CAD build for the part. Positions are in the model's coordinates, mm. Face numbers are marked on the shaded views. Give positions to 0.01 mm unless a question says otherwise; leave off trailing zeros. Order: outer loops, then holes, each group sorted by start corner. A loop starts at its lowest first (then second) coordinate and runs counter-clockwise, first axis right, second up.
```python
from build123d import *

# Parameters (mm, degrees)
F0_W     = 70.3723412007
F0_H     = 39.6034847945
F2_DEPTH = 9.5
F1_R     = 2.35
F3_DEPTH = 8


# Not quite as in the source:
# - the program builds the solid bodies; features that only make, move or delete a surface that nothing else refers to are left out


with BuildPart() as f2:
    # F0 (on Top) → F2 (new body)
    with BuildSketch(Plane.XY):
        with Locations((-25.7422635332, 26.3515496626)):
            Rectangle(F0_W, F0_H)
    extrude(amount=F2_DEPTH)

    # F1 (on face) → F3 (cut)
    with BuildSketch(Plane.XY):
        with BuildLine():
            ThreePointArc((-26.0081397088, 24.315958029), (-26.0169226605, 24.8283618655), (-26.0432611967, 25.3401636957))
            ThreePointArc((-26.0432611967, 25.3401636957), (-29.6543131579, 29.4708098057), (-30.4048881867, 34.9057496103))
            ThreePointArc((-30.4048881867, 34.9057496103), (-54.7680712155, 18.5828288025), (-26.0081397088, 24.315958029))
        make_face()
        with BuildLine():
            ThreePointArc((-18.4289942121, 24.2039844017), (-10.2782880331, 12.4173582289), (0.4453969671, 21.9232063115))
            ThreePointArc((0.4453969671, 21.9232063115), (0.1704350534, 24.2013451557), (-0.6386587183, 26.348642973))
            ThreePointArc((-0.6386587183, 26.348642973), (-4.6497239534, 27.6234855531), (-6.8365136406, 31.2195693659))
            ThreePointArc((-6.8365136406, 31.2195693659), (-9.2433206047, 31.4975310038), (-11.6428466394, 31.1624828835))
            ThreePointArc((-11.6428466394, 31.1624828835), (-14.0873300566, 26.758138344), (-18.4289942121, 24.2039844017))
        make_face()
        with BuildLine():
            ThreePointArc((-26.0432611967, 25.3401636957), (-22.3553467612, 23.9731105992), (-18.4289942121, 24.2039844017))
            ThreePointArc((-18.4289942121, 24.2039844017), (-15.9845107949, 28.6083289412), (-11.6428466394, 31.1624828835))
            ThreePointArc((-11.6428466394, 31.1624828835), (-11.436389736, 32.2945759735), (-11.3672378186, 33.4432609737))
            ThreePointArc((-11.3672378186, 33.4432609737), (-20.2088389756, 42.9901322485), (-30.4048881867, 34.9057496103))
            ThreePointArc((-30.4048881867, 34.9057496103), (-27.3555998695, 30.5189557333), (-26.0432611967, 25.3401636957))
        make_face()
        with Locations((-20.9422378186, 33.4432609737)):
            Circle(F1_R, mode=Mode.SUBTRACT)
        with BuildLine():
            ThreePointArc((-6.8365136406, 31.2195693659), (-3.2130730762, 29.4515061375), (-0.6386587183, 26.348642973))
            ThreePointArc((-0.6386587183, 26.348642973), (3.4064099368, 28.2070418834), (5.0577621814, 32.340958029))
            ThreePointArc((5.0577621814, 32.340958029), (-1.5054185479, 38.3144685099), (-6.8365136406, 31.2195693659))
        make_face()
        with BuildLine():
            ThreePointArc((-30.4048881867, 34.9057496103), (-29.6543131579, 29.4708098057), (-26.0432611967, 25.3401636957))
            ThreePointArc((-26.0432611967, 25.3401636957), (-27.3555998695, 30.5189557333), (-30.4048881867, 34.9057496103))
        make_face()
        with BuildLine():
            ThreePointArc((-11.6428466394, 31.1624828835), (-15.9845107949, 28.6083289412), (-18.4289942121, 24.2039844017))
            ThreePointArc((-18.4289942121, 24.2039844017), (-14.0873300566, 26.758138344), (-11.6428466394, 31.1624828835))
        make_face()
        with Locations((-20.9422378186, 33.4432609737)):
            Circle(F1_R)
        with BuildLine():
            ThreePointArc((-6.8365136406, 31.2195693659), (-4.6497239534, 27.6234855531), (-0.6386587183, 26.348642973))
            ThreePointArc((-0.6386587183, 26.348642973), (-3.2130730762, 29.4515061375), (-6.8365136406, 31.2195693659))
        make_face()
    extrude(amount=F3_DEPTH, mode=Mode.SUBTRACT)


solid = f2.part
```
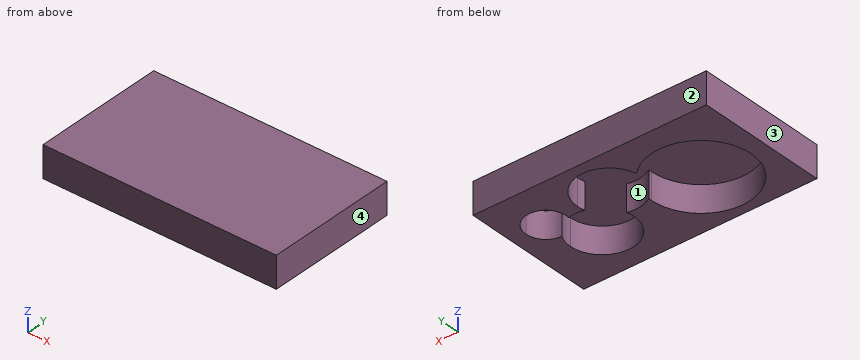
Item 1: Two-plate mould, pull along X, no slides. Class the marked faces 1, 2, 3 and 4: released by +X, released by -X, zero draft, split by the parting line, or undercut.
Item 2: Slice it at C-C (y = 41). Give the cut face in (x, z), and give its area (3 significant figures).
Item 3: Slice it at B-B (x = -43). Give the cut face in (y, z), and give its area (3 significant figures).
Item 4: Slice it at A-A (z = 1.75). Give the cut face in (x, y) (3 decimals), and give its area (3 significant figures).
Item 5: Wall check: L1, parallel to X at y = 25, z = 3; L2, parallel to X at y = 19, z = 0.5; L3, parallel to Z at x = -4, y = 28. Give the ranges that are in metal, low to high.
Item 6: Slice it at D-D (y = 16). Give the cut face in (x, z), and give its area (3 significant figures).
Item 7: Drop a flat-ended pin along its axis: pin 1 Ø1 at (x, y) = (-52.5, 26.5) entering from -Z. Give the stop position or say it passes through.
A:
1. face 1: undercut
1. face 2: zero draft
1. face 3: released by -X
1. face 4: released by +X
2. outline: (-60.93, 0) - (-26.82, 0) - (-26.82, 8) - (-15.06, 8) - (-15.06, 0) - (9.44, 0) - (9.44, 9.5) - (-60.93, 9.5) - close
2. area: 574 mm2
3. outline: (6.55, 0) - (9.5, 0) - (9.5, 8) - (39.13, 8) - (39.13, 0) - (46.15, 0) - (46.15, 9.5) - (6.55, 9.5) - close
3. area: 139 mm2
4. outline: (-60.928, 6.55) - (9.444, 6.55) - (9.444, 46.153) - (-60.928, 46.153) - close; hole (-30.405, 34.906) arc R14.951 ccw (long way) to (-26.043, 25.34) arc R9.575 ccw to (-18.429, 24.204) arc R9.575 ccw (long way) to (-0.639, 26.349) arc R6 ccw (long way) to (-6.837, 31.22) arc R9.575 ccw to (-11.643, 31.162) arc R9.575 ccw (long way) to start
4. area: 1,440 mm2
5. L1: x = -60.93 to -55.9, -26.02 to -25.46, -0.06 to 9.44
5. L2: x = -60.93 to -54.93, -26.99 to -18.25, -0.01 to 9.44
5. L3: z = 8 to 9.5
6. outline: (-60.93, 0) - (-53.38, 0) - (-53.38, 8) - (-28.53, 8) - (-28.53, 0) - (-16.65, 0) - (-16.65, 8) - (-1.61, 8) - (-1.61, 0) - (9.44, 0) - (9.44, 9.5) - (-60.93, 9.5) - close
6. area: 349 mm2
7. pin 1: stops at z = 8
